```python
from build123d import *

# Parameters (mm, degrees)
F0_R         = 2
F1_DEPTH     = 1.5
F2_R         = 2
F3_DEPTH     = 6.5
F4_SIZE      = 1
F5_T1_DEPTH  = 27.5
F5_T6_DEPTH  = 16.75
F5_S7_R      = 5.25
F5_T8_DEPTH  = 10
F5_T12_DEPTH = 16.75
F5_S13_R     = 5.25
F5_T14_DEPTH = 10
F6_SIZE      = 0.5
F7_R         = 0.5
F8_T1_DEPTH  = 12.35
F8_T4_ANGLE  = 90
F8_T6_ANGLE  = 90


# Not quite as in the source:
# - a fillet or chamfer that OpenCascade refuses, or shapes differently, is made with other operations: its cross-section is extruded or revolved along the edge and cut away or added


with BuildPart() as f1:
    # F0 (on Top) → F1 (new body)
    with BuildSketch(Plane.XY):
        with BuildLine():
            ThreePointArc((38.3721691668, 6.4511308521), (33.1221691668, 11.7011308521), (27.8721691668, 6.4511308521))
            Line((27.8721691668, 6.4511308521), (27.8721691668, -5.5488691479))
            ThreePointArc((27.8721691668, -5.5488691479), (33.1221691668, -10.7988691479), (38.3721691668, -5.5488691479))
            Line((38.3721691668, -5.5488691479), (38.3721691668, 6.4511308521))
        make_face()
        with Locations((33.1221691668, -3.5488691479)):
            Circle(F0_R, mode=Mode.SUBTRACT)
        with Locations((33.1221691668, 4.4511308521)):
            Circle(F0_R, mode=Mode.SUBTRACT)
    extrude(amount=F1_DEPTH)

    # F2 (on face) → F3 (join)
    with BuildSketch(Plane.XY.offset(1.5)):
        with BuildLine():
            Line((38.3721691668, -5.5488691479), (38.3721691668, 6.4511308521))
            ThreePointArc((38.3721691668, 6.4511308521), (36.834479768, 10.1634414533), (33.1221691668, 11.7011308521))
            Line((33.1221691668, 11.7011308521), (23.1221691668, 11.7011308521))
            Line((23.1221691668, 11.7011308521), (23.1221691668, -10.7988691479))
            Line((23.1221691668, -10.7988691479), (33.1221691668, -10.7988691479))
            ThreePointArc((33.1221691668, -10.7988691479), (36.834479768, -9.2611797491), (38.3721691668, -5.5488691479))
        make_face()
        with Locations((33.1221691668, -3.5488691479)):
            Circle(F2_R, mode=Mode.SUBTRACT)
        with Locations((33.1221691668, 4.4511308521)):
            Circle(F2_R, mode=Mode.SUBTRACT)
    extrude(amount=F3_DEPTH)

    # F4
    f4_edges = [f1.edges().sort_by_distance(p)[0] for p in [
        (27.872169, 0.451131, 0),
        (38.372169, 0.451131, 0),
        (33.122169, 11.701131, 0),
        (33.122169, -10.798869, 0),
    ]]
    chamfer(f4_edges, length=F4_SIZE)

    # F5: fillet of radius 1 on 3 edges, made by hand

    # F5_s2 → F5_t1 (cut)
    with BuildSketch(Plane.XZ.offset(-14.2011308521)):
        with BuildLine():
            ThreePointArc((24.1221691668, 1.5), (23.4150623856, 1.7928932188), (23.1221691668, 2.5))
            Line((23.1221691668, 2.5), (23.1221691668, 1.5))
            Line((23.1221691668, 1.5), (24.1221691668, 1.5))
        make_face()
    extrude(amount=F5_T1_DEPTH, mode=Mode.SUBTRACT)


with BuildPart() as f5_tool4:
    # F5_s5 → F5_t6 (new body)
    with BuildSketch(Plane.YZ.offset(37.3721691668)):
        with BuildLine():
            ThreePointArc((10.7011308521, 1.5), (11.4082376333, 1.7928932188), (11.7011308521, 2.5))
            Line((11.7011308521, 2.5), (11.7011308521, 1.5))
            Line((11.7011308521, 1.5), (10.7011308521, 1.5))
        make_face()
    extrude(amount=-F5_T6_DEPTH)

    # F5_s7 → F5_t8 (cut, symmetric)
    with BuildSketch(Plane.XY.offset(2)):
        with Locations((33.1221691668, 6.4511308521)):
            Circle(F5_S7_R)
    extrude(amount=F5_T8_DEPTH, both=True, mode=Mode.SUBTRACT)


with BuildPart() as f1_1:
    add(f1.part)

    # F5_t3: cut F5_tool4
    add(f5_tool4.part, mode=Mode.SUBTRACT)


with BuildPart() as f5_tool10:
    # F5_s11 → F5_t12 (new body)
    with BuildSketch(Plane.YZ.offset(20.6221691668)):
        with BuildLine():
            ThreePointArc((-9.7988691479, 1.5), (-10.5059759291, 1.7928932188), (-10.7988691479, 2.5))
            Line((-10.7988691479, 2.5), (-10.7988691479, 1.5))
            Line((-10.7988691479, 1.5), (-9.7988691479, 1.5))
        make_face()
    extrude(amount=F5_T12_DEPTH)

    # F5_s13 → F5_t14 (cut, symmetric)
    with BuildSketch(Plane.XY.offset(2)):
        with Locations((33.1221691668, -5.5488691479)):
            Circle(F5_S13_R)
    extrude(amount=F5_T14_DEPTH, both=True, mode=Mode.SUBTRACT)


with BuildPart() as f1_2:
    add(f1_1.part)

    # F5_t9: cut F5_tool10
    add(f5_tool10.part, mode=Mode.SUBTRACT)

    # F6
    f6_edges = [f1_2.edges().sort_by_distance(p)[0] for p in [
        (28.122169, 11.701131, 8),
        (38.372169, 0.451131, 8),
        (36.83448, -9.26118, 8),
        (36.83448, 10.163441, 8),
        (28.122169, -10.798869, 8),
    ]]
    chamfer(f6_edges, length=F6_SIZE)

    # F7
    f7_edges = [f1_2.edges().sort_by_distance(p)[0] for p in [
        (31.122169, -3.548869, 0),
        (31.122169, 4.451131, 0),
    ]]
    fillet(f7_edges, radius=F7_R)

    # F8: fillet of radius 2.54 on 2 edges, made by hand

    # F8_s2 → F8_t1 (cut)
    with BuildSketch(Plane.XY.offset(1.5)):
        with BuildLine():
            ThreePointArc((25.6621691668, 11.7011308521), (23.8661179426, 10.9571820763), (23.1221691668, 9.1611308521))
            Line((23.1221691668, 9.1611308521), (23.1221691668, 11.7011308521))
            Line((23.1221691668, 11.7011308521), (25.6621691668, 11.7011308521))
        make_face()
        with BuildLine():
            ThreePointArc((25.6621691668, -10.7988691479), (23.8661179426, -10.0549203721), (23.1221691668, -8.2588691479))
            Line((23.1221691668, -8.2588691479), (23.1221691668, -10.7988691479))
            Line((23.1221691668, -10.7988691479), (25.6621691668, -10.7988691479))
        make_face()
    extrude(amount=F8_T1_DEPTH, mode=Mode.SUBTRACT)

    # F8_s3 → F8_t4 (revolve, cut)
    with BuildSketch(Plane.YZ.offset(25.6621691668)):
        with BuildLine():
            ThreePointArc((-9.7988691479, 1.5), (-10.5059759291, 1.7928932188), (-10.7988691479, 2.5))
            Line((-10.7988691479, 2.5), (-10.7988691479, 1.5))
            Line((-10.7988691479, 1.5), (-9.7988691479, 1.5))
        make_face()
    revolve(axis=Axis((25.6621691668, -8.2588691479, 1.5), (0, 0, -1)), revolution_arc=F8_T4_ANGLE, mode=Mode.SUBTRACT)

    # F8_s5 → F8_t6 (revolve, cut)
    with BuildSketch(Plane.XZ.offset(-9.1611308521)):
        with BuildLine():
            ThreePointArc((24.1221691668, 1.5), (23.4150623856, 1.7928932188), (23.1221691668, 2.5))
            Line((23.1221691668, 2.5), (23.1221691668, 1.5))
            Line((23.1221691668, 1.5), (24.1221691668, 1.5))
        make_face()
    revolve(axis=Axis((25.6621691668, 9.1611308521, 1.5), (0, 0, -1)), revolution_arc=F8_T6_ANGLE, mode=Mode.SUBTRACT)


solid = f1_2.part
```
Work out the finished part from the listing and answer in its coordinate system (mm). A direction names the side the tool comes from. Round coordinates to 2 decimals unless told otherwise and drop trailing zeros. Write each loop counter-clockwise with the first axis right and the second up, starting at its lowest first coordinate (ties: lowest second). Pieces come first, ordered by that corner, then holes. Notation, with made-up numbers: (70, -32.75) - (87, -32.75) arc R23 cw to (87, 5.25) - close; hole circle Ø9 at (42.5, 61). An arc over 180 degrees is marked (long way). Return JSON: item names as keys, results as strings. Group by question number.
Q1. The part is cut by section C-C on x = 31.75. Count the separate pieces of the cut face and the enclosed holes in it, then the cut area to 3 significant figures.
Q2. Find the intervals of material crossed by L1, parallel to Y at x = 32.5, z = 5.25; L2, parallel to Z at x = 25.5, y = 1.5; L3, parallel to Y at x = 31.75, z = 1.5, in increasing order.
Q3. The mould has two halves that part along Y. Classify faces 3 (the flat face through (29, -10.799, 5)), 4 (the cylindrical face through (32.862, -1.566, 4.198)), 5 (the flat face through (37.865, 0.367, 0.493)): released by +Y, released by -Y, zero draft, split by the parting line, or undercut.
Q4. Each of these flat-tipped pins is pushed along its axis until it touches: pin 1 Ø2 at (x, z) = (24.5, 4.5) entering from -Y; pin 2 Ø1.5 at (y, z) = (-7.5, 5) entering from +X. Where does it stop, or does it pass through?
Q5. The part is cut by section B-B on z = 6.5. Write down the section's boundary in (x, y).
Q6. For faces 1 (the cylindrical face through (28.511, -10.498, 1.785)), 2 (the conical face through (33.2, 10.9, 0.2)), determine the directions among +Z, -Z, +X, -X, +Y, -Y from which every point of the face is accessible in a straight line to the end or side of a thin tool.
Q7. The part is cut by section A-A on x = 27.5. Write down the section's boundary in (y, z), then the cut area to 3 significant figures.
Q8. The part is cut by section D-D on z = 1.75. Write down the section's boundary in (x, y), then the cut area to 3 significant figures.
Solved:
{
 "1": {"separate pieces": "3", "enclosed holes": "0", "area": "131 mm²"},
 "2": {"L1": "-10.8 to -5.45, -1.65 to 2.55, 6.35 to 11.7", "L2": "1.5 to 8", "L3": "-10.62 to -5, -2.09 to 3, 5.91 to 11.52"},
 "3": {"face 3": "released by -Y", "face 4": "undercut", "face 5": "zero draft"},
 "4": {"pin 1": "y = -10.79", "pin 2": "x = 38.23"},
 "5": {"outline": "(23.12, -8.26) arc R2.54 ccw to (25.66, -10.8) - (33.12, -10.8) arc R5.25 ccw to (38.37, -5.55) - (38.37, 6.45) arc R5.25 ccw to (33.12, 11.7) - (25.66, 11.7) arc R2.54 ccw to (23.12, 9.16) - close; hole circle Ø4 at (33.12, -3.55); hole circle Ø4 at (33.12, 4.45)"},
 "6": {"face 1": "-Z, -X, -Y", "face 2": "-Z, +Y"},
 "7": {"outline": "(-10.8, 2.5) arc R1 ccw to (-9.8, 1.5) - (10.7, 1.5) arc R1 ccw to (11.7, 2.5) - (11.7, 7.5) - (11.2, 8) - (-10.3, 8) - (-10.8, 7.5) - close", "area": "146 mm²"},
 "8": {"outline": "(23.46, -8.26) arc R2.2 ccw to (25.66, -10.46) - (31.27, -10.46) arc R5.25 ccw to (38.37, -5.55) - (38.37, 6.45) arc R5.25 ccw to (31.27, 11.36) - (25.66, 11.36) arc R2.2 ccw to (23.46, 9.16) - close; hole circle Ø4 at (33.12, -3.55); hole circle Ø4 at (33.12, 4.45)", "area": "291 mm²"}
}
